Input: part model. Units: mm. Frame: model coordinates. Face numbers are marked on the shaded views. A direction names the side the tool comes from. Coordinates: 2 decimals unless noted, no trailing zeros. Loops run counter-clockwise (first coordinate to the right, second up) from the corner with the lowest first, then second, coordinate; pieces in that order, holes last. Notation, with made-up numbers: (-32, 21) -> (-19, 21) arc R23 ccw to (-19, 47) -> close; hole circle Ø10 at (72.5, -4). An arc over 180 degrees is marked (long way). Put each result on its own line as item: value. Start each with the question number.
1) Cut plane D-D (x = 2.75). Return the cut outline in (y, z), plus the area to 3 significant figures.
2) Contact query for flat-ended pins moving along their axis: P1, Ø1.3, axis at y = -1, z = 16.5, coming from the -X side; P2, Ø3, axis at x = -9.5, y = 17, coming from the +Z side; P3, Ø4, axis at x = -5, z = 20.5, coming from the +Y side; P4, Ø4, axis at x = 1, z = 18, coming from the +Y side. Output: stop coordinate, or through.
3) Cut plane A-A (x = -3.5). Return the cut outline in (y, z), plus the area to 3 significant figures.
4) Material intervals for L1, parallel to Y at x = -14, z = 32; L2, parallel to Y at x = -5.25, z = 17.5; L3, parallel to Y at x = 4.25, z = 36.5, sorted ascending.
5) Set-up query: the marked faces 1, 2 and 3. Return all of +Z, -Z, +X, -X, +Y, -Y with unobstructed straight access to the full face (end or side cutting, diameter ignored); none if empty.
6) Cut plane C-C (x = -15.5). Return the cut outline in (y, z), plus the area to 3 significant figures.
from build123d import *

# Parameters (mm, degrees)
F1_DEPTH = 50
F2_R     = 5
F3_R     = 2.5
F4_R     = 0.49999


# Not quite as in the source:
# - a fillet or chamfer is up to 0.001 mm smaller than in the source, because OpenCascade refuses the exact size


with BuildPart() as f1:
    # F0 (on Top) → F1 (new body)
    with BuildSketch(Plane.XY):
        with BuildLine():
            Line((7, 2.5), (10, 2.5))
            ThreePointArc((10, 2.5), (4.1421356237, 16.6421356237), (-10, 22.5))
            Line((-10, 22.5), (-20, 22.5))
            Line((-20, 22.5), (-20, 19.5))
            Line((-20, 19.5), (-10, 19.5))
            ThreePointArc((-10, 19.5), (2.0208152802, 14.5208152802), (7, 2.5))
        make_face()
        Polygon((-10, -2.5), (10, -2.5), (10, 2.5), (7, 2.5), (-10, 2.5), align=None)
    extrude(amount=F1_DEPTH)

    # F2
    f2_edges = [f1.edges().sort_by_distance(p)[0] for p in [
        (7, 2.5, 25),
    ]]
    fillet(f2_edges, radius=F2_R)

    # F3
    f3_edges = [f1.edges().sort_by_distance(p)[0] for p in [
        (-20, 22.5, 25),
        (-10, 2.5, 25),
    ]]
    fillet(f3_edges, radius=F3_R)

    # F4 (radius 0.5 in the source; OpenCascade refuses exactly that, so slightly less here)
    f4_edges = [f1.edges().sort_by_distance(p)[0] for p in [
        (-20, 19.5, 25),
    ]]
    fillet(f4_edges, radius=F4_R)


solid = f1.part
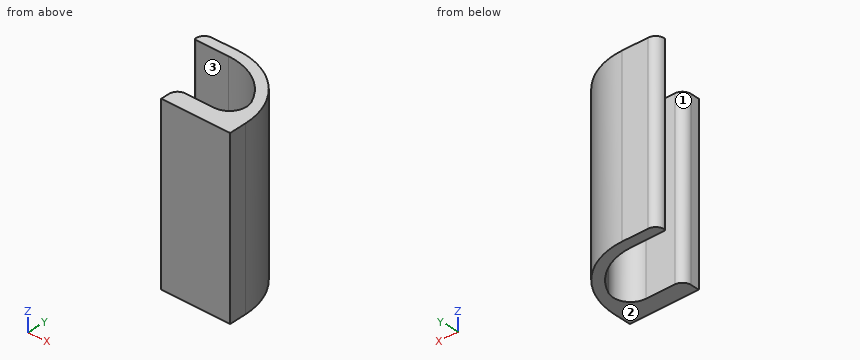
Results found:
1. outline: (-2.5, 0) -> (2.85, 0) -> (2.85, 50) -> (-2.5, 50) -> close; (13.74, 0) -> (17.91, 0) -> (17.91, 50) -> (13.74, 50) -> close
1. area: 476 mm2
2. P1: stops at x = -10
2. P2: passes through
2. P3: stops at y = 22.27
2. P4: stops at y = 20.36
3. outline: (-2.5, 0) -> (2.5, 0) -> (2.5, 50) -> (-2.5, 50) -> close; (18.21, 0) -> (21.41, 0) -> (21.41, 50) -> (18.21, 50) -> close
3. area: 410 mm2
4. L1: y = 19.5 to 22.5
4. L2: y = -2.5 to 2.5, 18.82 to 21.93
4. L3: y = -2.5 to 3.78, 11.77 to 16.53
5. face 1: +Z, -Z, -X
5. face 2: -Z, +X, -X, +Y, -Y
5. face 3: +Z, -Z, -X, -Y
6. outline: (19.5, 0) -> (22.5, 0) -> (22.5, 50) -> (19.5, 50) -> close
6. area: 150 mm2
